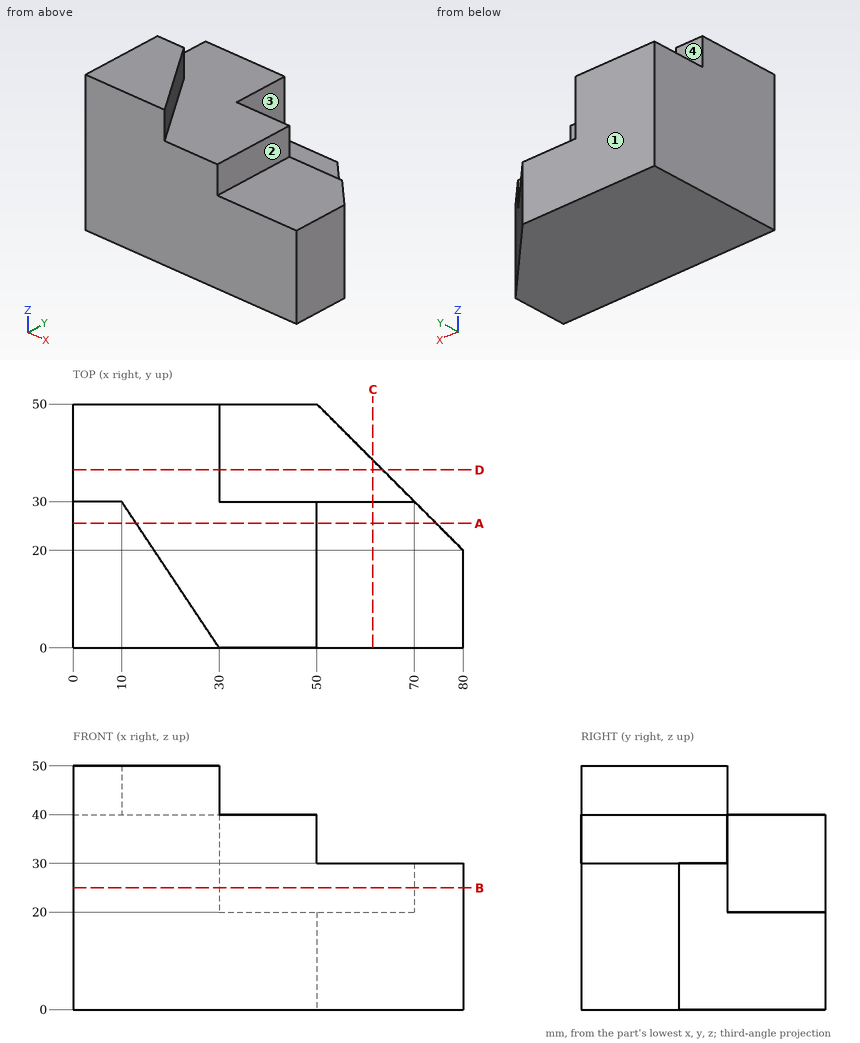
The drawing under review shows one solid part. Ordinate dimensions are in mm from its lowest x, y, z. A direction names the side the tool comes from. Round coordinates to 2 decimals unless told otherwise and drop trailing zeros. Loops run counter-clockwise (first coordinate to the right, second up) from the corner with the lowest first, then second, coordinate; pieces in that order, holes last. Notation, with made-up numbers: (66, -9.75) -> (86, -9.75) arc R17 cw to (86, 19.25) -> close; hole circle Ø8 at (-32, 77.5). An arc over 180 degrees is marked (long way). Answer in a Markdown table with one row per item.
1) Wall thickness on line 1 along X through (y, z) = (46.5, 38); line 2 along Z through (x, y) = (49, 11.5); line 3 along Z through (x, y) = (47.5, 38): over which ranges is each line inside the solid? List them lowest first.
Taken from the geometry:
| item | result |
|---|---|
| line 1 | x = 0 to 30 |
| line 2 | z = 0 to 40 |
| line 3 | z = 0 to 20 |
2) Consider section B-B, the plane z = 25. Write out the cut boundary in (x, y), plus the area to 3 significant figures.
Taken from the geometry:
| item | result |
|---|---|
| outline | (0, 0) -> (80, 0) -> (80, 20) -> (70, 30) -> (30, 30) -> (30, 50) -> (0, 50) -> close |
| area | 2,950 mm² |
3) Consider section C-C, the plane x = 61.5. Write out the cut boundary in (y, z), plus the area to 3 significant figures.
Taken from the geometry:
| item | result |
|---|---|
| outline | (0, 0) -> (38.5, 0) -> (38.5, 20) -> (30, 20) -> (30, 30) -> (0, 30) -> close |
| area | 1,070 mm² |
4) For pin 1 Ø8 at (y, z) = (8, 36.5) entering from +X; pin 2 Ø6 at (x, z) = (48, 31.5) entering from +Y; pin 3 Ø2 at (x, y) = (32, 36) entering from +Z, all flat-tipped, find the tip position at first contact; note any pin that passes through.
Taken from the geometry:
| item | result |
|---|---|
| pin 1 | stops at x = 50 |
| pin 2 | stops at y = 30 |
| pin 3 | stops at z = 20 |
5) Consider section D-D, the plane y = 36.5. Write out the cut boundary in (x, z), plus the area to 3 significant figures.
Taken from the geometry:
| item | result |
|---|---|
| outline | (0, 0) -> (63.5, 0) -> (63.5, 20) -> (30, 20) -> (30, 40) -> (0, 40) -> close |
| area | 1,870 mm² |
6) Tool access review of the marked faces 1, 2, 3 and 4: name each direction out of +Z, -Z, +X, -X, +Y, -Y from which nothing blocks a thin tool from reaching the whole face with its end or side.
Taken from the geometry:
| item | result |
|---|---|
| face 1 | +Z, -Z, +X, -X, +Y |
| face 2 | +Z, +X, +Y, -Y |
| face 3 | +Z, +X, +Y |
| face 4 | +Z, +X, -X, +Y |
7) Consider section A-A, the plane y = 25.5. Write out the cut boundary in (x, z), plus the area to 4 significant figures.
Taken from the geometry:
| item | result |
|---|---|
| outline | (0, 0) -> (74.5, 0) -> (74.5, 30) -> (50, 30) -> (50, 40) -> (13, 40) -> (13, 50) -> (0, 50) -> close |
| area | 2,865 mm² |
